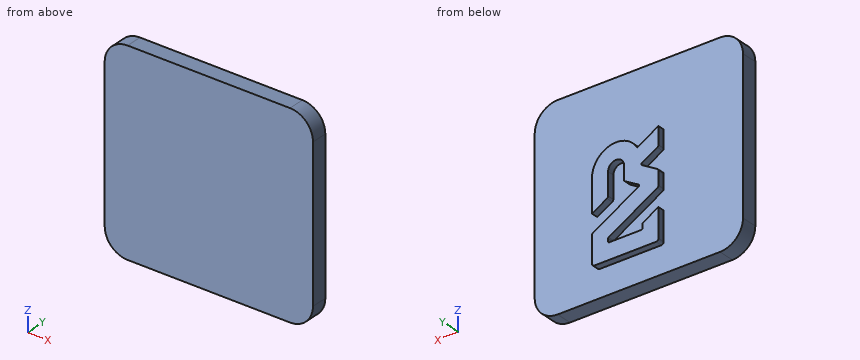
from build123d import *

# Parameters (mm, degrees)
SKETCH1_W           = 90.757028804
SKETCH1_H           = 85.620479834
BOSS_EXTRUDE1_DEPTH = 10
SKETCH2_W           = 90.757028804
SKETCH2_H           = 85.620479834
CUT_EXTRUDE1_DEPTH  = 3
FILLET3_R           = 10
FILLET4_R           = 0.5


with BuildPart() as part:
    # Sketch1 → Boss-Extrude1 (new body)
    with BuildSketch(Plane(origin=(0, 0, 0), x_dir=(1, 0, 0), z_dir=(0, 1, 0))):
        with Locations((50.879550114, -25.035867198)):
            Rectangle(SKETCH1_W, SKETCH1_H)
    extrude(amount=BOSS_EXTRUDE1_DEPTH)

    # Sketch2 → Cut-Extrude1 (cut)
    with BuildSketch(Plane(origin=(0, 10, 0), x_dir=(1, 0, 0), z_dir=(0, 1, 0))):
        with Locations((50.879550114, -25.035867198)):
            Rectangle(SKETCH2_W, SKETCH2_H)
        with BuildLine():
            ThreePointArc((67.972256686, 6.083430281), (68.679363467, 5.790537062), (68.972256686, 5.083430281))
            Line((68.972256686, 5.083430281), (68.972256686, -6.33921945))
            ThreePointArc((68.972256686, -6.33921945), (68.83828209, -6.83921945), (68.472256686, -7.205244854))
            Line((68.472256686, -7.205244854), (48.722256686, -18.60791267))
            ThreePointArc((48.722256686, -18.60791267), (48.472256686, -19.040925372), (48.722256686, -19.473938074))
            Line((48.722256686, -19.473938074), (54.972256686, -23.082377257))
            Line((54.972256686, -23.082377257), (54.972256686, -29.289636678))
            ThreePointArc((54.972256686, -29.289636678), (58.472256686, -32.789636678), (61.972256686, -29.289636678))
            Line((61.972256686, -29.289636678), (61.972256686, -19.618275642))
            ThreePointArc((61.972256686, -19.618275642), (62.106231282, -19.118275642), (62.472256686, -18.752250238))
            Line((62.472256686, -18.752250238), (68.972256686, -14.999473488))
            Line((68.972256686, -14.999473488), (68.972256686, -29.289636678))
            ThreePointArc((68.972256686, -29.289636678), (61.12912537, -39.447936181), (49.316818821, -34.430449599))
            Line((49.316818821, -34.430449599), (47.972256686, -35.20673291))
            Line((47.972256686, -35.20673291), (40.034434513, -39.789636678))
            Line((40.034434513, -39.789636678), (40.034434513, -32.284083179))
            ThreePointArc((40.034434513, -32.284083179), (40.168409109, -31.784083179), (40.534434513, -31.418057775))
            Line((40.534434513, -31.418057775), (47.972256686, -27.123829141))
            Line((47.972256686, -27.123829141), (40.534434513, -22.829600507))
            ThreePointArc((40.534434513, -22.829600507), (40.168409109, -22.463575103), (40.034434513, -21.963575103))
            Line((40.034434513, -21.963575103), (40.034434513, -16.118275642))
            ThreePointArc((40.034434513, -16.118275642), (40.168409109, -15.618275642), (40.534434513, -15.252250238))
            Line((40.534434513, -15.252250238), (61.722256686, -3.019455402))
            ThreePointArc((61.722256686, -3.019455402), (61.905269388, -2.8364427), (61.972256686, -2.5864427))
            Line((61.972256686, -2.5864427), (61.972256686, -1.416569719))
            ThreePointArc((61.972256686, -1.416569719), (61.825810077, -1.063016329), (61.472256686, -0.916569719))
            Line((61.472256686, -0.916569719), (47.534434513, -0.916569719))
            ThreePointArc((47.534434513, -0.916569719), (47.180881122, -1.063016329), (47.034434513, -1.416569719))
            Line((47.034434513, -1.416569719), (47.034434513, -3.127894585))
            ThreePointArc((47.034434513, -3.127894585), (46.967447214, -3.377894585), (46.784434513, -3.560907287))
            Line((46.784434513, -3.560907287), (40.034434513, -7.458021604))
            Line((40.034434513, -7.458021604), (40.034434513, -6.916569719))
            Line((40.034434513, -6.916569719), (40.034434513, 5.083430281))
            ThreePointArc((40.034434513, 5.083430281), (40.327327731, 5.790537062), (41.034434513, 6.083430281))
            Line((41.034434513, 6.083430281), (67.972256686, 6.083430281))
        make_face(mode=Mode.SUBTRACT)
    extrude(amount=-CUT_EXTRUDE1_DEPTH, mode=Mode.SUBTRACT)

    # Fillet3
    fillet3_edges = [part.edges().sort_by_distance(p)[0] for p in [
        (5.501035712, 3.5, -17.774372719),
        (96.258064516, 3.5, -17.774372719),
        (96.258064516, 3.5, 67.846107115),
        (5.501035712, 3.5, 67.846107115),
    ]]
    fillet(fillet3_edges, radius=FILLET3_R)

    # Fillet4
    fillet4_edges = [part.edges().sort_by_distance(p)[0] for p in [
        (47.972256686, 8.5, 27.123829141),
        (54.972256686, 8.5, 23.082377257),
    ]]
    fillet(fillet4_edges, radius=FILLET4_R)


solid = part.part
CAD build for the part. Positions are in the model's coordinates, mm. Round coordinates to 2 decimals unless told otherwise and drop trailing zeros. Order: outer loops, then holes, each group sorted by start corner. A loop starts at its lowest first (then second) coordinate and runs counter-clockwise, first axis right, second up. Notation, with made-up numbers: (-23.75, 30.25) - (-19.75, 30.25) arc R29 cw to (-19.75, 57.25) - close; hole circle Ø7 at (80, 76.5). An arc over 180 degrees is marked (long way). Return JSON: item names as keys, results as strings.
(1) Cut at B-B (x = 22.5). Give the cut face in (y, z), then the cut area to 3 significant figures.
Answer key:
{"outline": "(0, -17.77) - (7, -17.77) - (7, 67.85) - (0, 67.85) - close", "area": "599 mm^2"}
(2) Cut at D-D (z = 44). Give the cut face in (x, y).
Answer key:
{"outline": "(5.5, 0) - (96.26, 0) - (96.26, 7) - (5.5, 7) - close"}
(3) Cut at C-C (x = 52). Give the cut face in (y, z).
Answer key:
{"outline": "(0, -17.77) - (7, -17.77) - (7, -6.08) - (10, -6.08) - (10, 0.92) - (7, 0.92) - (7, 8.63) - (10, 8.63) - (10, 16.72) - (7, 16.72) - (7, 21.37) - (10, 21.37) - (10, 37.56) - (7, 37.56) - (7, 67.85) - (0, 67.85) - close"}
(4) Wall check: probe 1 along Y at (x, z) = (75, 4); probe 2 along X at (y, z) = (7.5, -2.5); probe 3 along X at (y, z) = (2, 64). Give the ranges that are in metal, low to high. Write a range as from..to.
Answer key:
{"probe 1": "y = 0..7", "probe 2": "x = 40.03..68.97", "probe 3": "x = 7.62..94.14"}
(5) Cut at A-A (z = -0.5). Give the cut face in (x, y), then the cut area to 3 significant figures.
Answer key:
{"outline": "(5.5, 0) - (96.26, 0) - (96.26, 7) - (68.97, 7) - (68.97, 10) - (40.03, 10) - (40.03, 7) - (5.5, 7) - close", "area": "722 mm^2"}
(6) Pin check, flat tips, straight feed: pin 1 Ø2.5 at (x, y) = (56.5, 9) entering from +Z; pin 2 Ø1.5 at (x, z) = (32.5, 34) entering from +Y; pin 3 Ø0.9 at (y, z) = (9, 2) entering from -X; pin 4 Ø1.5 at (x, y) = (70, 8.5) entering from -Z. Stop position of each tip, or through.
Answer key:
{"pin 1": "stops at z = 39.76", "pin 2": "stops at y = 7", "pin 3": "stops at x = 40.03", "pin 4": "passes through"}
